For this review, take the finished solid that the model builds, in its own axes (mm). A direction names the side the tool comes from. Give positions to 0.01 mm unless a question says otherwise; leave off trailing zeros. Write each loop counter-clockwise with the first axis right and the second up, starting at its lowest first coordinate (ties: lowest second). Pieces come first, ordered by that corner, then holes. Notation, with made-up numbers: M -19,75 L 7,75 A17 ccw 7,104 Z; hole C 74,17 d10. An arc over 180 degrees is marked long. Use one line per item in the form item = value. Start each with the question number.
Q1. Consider section C-C on y = -39. Write out the cut boundary in (x, z).
Q2. Tool access review of faces 1 (the flat face through (-28, -25.4, 0)), 2 (the flat face through (-1, -13, -32.332)): name each direction out of +Z, -Z, +X, -X, +Y, -Y from which nothing blocks a thin tool from reaching the whole face with its end or side.
Q3. Consider section D-D on z = 21. Write out the cut boundary in (x, y), and give its area (3 significant figures).
Q4. Clearance check with flat-ended pins moving along their axes: pin 1 Ø19.5 at (x, z) = (5, -5.5) entering from -Y (3 decimals); pin 2 Ø12 at (y, z) = (-36.5, -17) entering from -X. State where each tip first meets the part, or that it passes through.
Q5. For probe 1 along Z at (x, y) = (0, -10.5); probe 2 along Y at (x, z) = (0, -25); probe 3 along Z at (x, y) = (0, -31), list the stretches that pass through material, from the lowest coordinate up. Write a range as [from, to].
Q6. Consider section A-A on x = 0. Write out the cut boundary in (y, z).
Q7. Mouldability with a two-part tool opening along X and no side actions: class faces 3 (the flat face through (-15, -50.8, -11)), 4 (the cylindrical face through (-14.6, -25.8, -11.2)), 5 (the cylindrical face through (-19.75, -37.92, -15.14)) as released by +X, released by -X, zero draft, split by the parting line, or undercut.
Q8. Consider section B-B on z = 0. Write out the cut boundary in (x, y), and give its area (3 significant figures).
```python
from build123d import *

# Parameters (mm, degrees)
F0_W     = 82.244918
F0_H     = 64.663574
F1_DEPTH = 25.4
F2_R     = 24.883851
F3_DEPTH = 25.4
F4_R     = 18.401021
F5_DEPTH = 127


with BuildPart() as f1:
    # F0 (on Front) → F1 (new body)
    with BuildSketch(Plane.XZ):
        Rectangle(F0_W, F0_H)
    extrude(amount=F1_DEPTH)

    # F2 (on face) → F3 (join)
    with BuildSketch(Plane.XZ.offset(25.4)):
        Circle(F2_R)
    extrude(amount=F3_DEPTH)

    # F4 (on face) → F5 (cut)
    with BuildSketch(Plane.XZ.offset(50.8)):
        Circle(F4_R)
    extrude(amount=-F5_DEPTH, mode=Mode.SUBTRACT)


solid = f1.part
```
Working result:
q1.outline = C 0,0 d49.77; hole C 0,0 d36.8
q2.face_1 = -Y
q2.face_2 = -Z, +X, -X, +Y, -Y
q3.outline = M -41.12,-25.4 L -13.35,-25.4 L -13.35,-50.8 L 13.35,-50.8 L 13.35,-25.4 L 41.12,-25.4 L 41.12,0 L -41.12,0 Z
q3.area = 2,770 mm²
q4.pin_1 = through
q4.pin_2 = -22.32
q5.probe_1 = [-32.33, -18.4], [18.4, 32.33]
q5.probe_2 = [-25.4, 0]
q5.probe_3 = [-24.88, -18.4], [18.4, 24.88]
q6.outline = M -50.8,-24.88 L -25.4,-24.88 L -25.4,-32.33 L 0,-32.33 L 0,-18.4 L -50.8,-18.4 Z; M -50.8,18.4 L 0,18.4 L 0,32.33 L -25.4,32.33 L -25.4,24.88 L -50.8,24.88 Z
q7.face_3 = zero draft
q7.face_4 = undercut
q7.face_5 = split by the parting line
q8.outline = M -41.12,-25.4 L -24.88,-25.4 L -24.88,-50.8 L -18.4,-50.8 L -18.4,0 L -41.12,0 Z; M 18.4,-50.8 L 24.88,-50.8 L 24.88,-25.4 L 41.12,-25.4 L 41.12,0 L 18.4,0 Z
q8.area = 1,480 mm²
